```python
from build123d import *

# Parameters (mm, degrees)
F1_DEPTH = 19
F3_D     = 9
F3_DEPTH = 30
F2_R     = 8.5
F2_R_2   = 7.5
F4_DEPTH = 10


with BuildPart() as f1:
    # F0 (on Front) → F1 (new body)
    with BuildSketch(Plane.XZ):
        Polygon((0, 10), (0, 0), (17, 0), align=None)
    extrude(amount=F1_DEPTH)

    # F3
    with Locations(Plane(origin=(4.37018, 0, 7.429306), x_dir=(0.861934, 0, -0.50702), z_dir=(0.50702, 0, 0.861934))):
        with Locations((4.79134, -9.5)):
            Hole(F3_D / 2, depth=F3_DEPTH)

    # F2 (on face) → F4 (join)
    with BuildSketch(Plane(origin=(4.37018, 0, 7.429306), x_dir=(0.861934, 0, -0.50702), z_dir=(0.50702, 0, 0.861934))):
        with Locations((4.79134, -9.5)):
            Circle(F2_R)
        with Locations((4.79134, -9.5)):
            Circle(F2_R_2, mode=Mode.SUBTRACT)
    extrude(amount=F4_DEPTH)


solid = f1.part
```
Design review of the part built by this model. Coordinates are the model's own, in mm. A direction names the side the tool comes from. Coordinates: 2 decimals unless noted, no trailing zeros. Write each loop counter-clockwise with the first axis right and the second up, starting at its lowest first coordinate (ties: lowest second). Pieces come first, ordered by that corner, then holes.
1) Add section A-A (y = -5.5). Write out the cut boundary in (x, z), plus the area to 3 significant figures.
2) Insertion check: pin 1 (1.5 mm diameter, centred on x = 18.5, z = 8.5, fed in from +Y); pin 2 (8 mm diameter, centred on y = -13.5, z = 15, fed in from -X); pin 3 (4 mm diameter, centred on x = 14, y = -10, fed in from +Z). Each pin has a flat end and moves straight along its axis. Give the tip position at first contact, or say it passes through.
3) Machinability: for faces 5 (the flat face through (5, 0, 3)), 6 (the flat face through (6.73, -0.92, 6.04)), which of the approach directions +Z, -Z, +X, -X, +Y, -Y give a long, thin tool a straight path to every point of the face, cutting with its end or side? Answer none if there is none.
4) Add section C-C (z = 2.25). State how many separate pieces and enclosed holes the cut face has, plus the area to 3 significant figures.
5) Mouldability with a two-part tool opening along Y and no side actions: class faces 1 (the flat face through (8.591, -14.395, 4.947)), 2 (the flat face through (12, -9, 0)), 3 (the flat face through (5, -19, 3)), 4 (the cylindrical face through (3.1, -8.15, 4.29)) as +Y half, -Y half, draft (parallel to the pull), parting line (faces both ways), or undercut.
6) Add section B-B (y = -12). Write out the cut boundary in (x, z) (3 decimals), plus the area to 3 significant figures.
7) To check wall thickness, follow L1, parallel to X at y = -8.5, z = 1.75 (3 decimals); L2, parallel to Y at x = 8.75, z = 6 (3 decimals); L3, parallel to X at y = -5.5, z = 3.25 (3 decimals). State the ranges of each line that lie inside material, in increasing order.
Check result:
1. outline: (0, 0) - (3.17, 0) - (6.72, 6.05) - (3.03, 8.22) - (8.1, 16.84) - (7.11, 17.42) - (2.04, 8.8) - (0, 10) - close; (7.95, 0) - (17, 0) - (14.96, 1.2) - (20.03, 9.82) - (19.04, 10.4) - (13.97, 1.78) - (10.28, 3.95) - close
1. area: 84.2 mm2
2. pin 1: stops at y = -3.58
2. pin 2: stops at x = 2.76
2. pin 3: stops at z = 3.01
3. face 5: +Z, -Z, +X, -X, +Y
3. face 6: none
4. separate pieces: 1
4. enclosed holes: 2
4. area: 192 mm2
5. face 1: undercut
5. face 2: draft
5. face 3: -Y half
5. face 4: undercut
6. outline: (0, 0) - (1.218, 0) - (5.275, 6.897) - (2.405, 8.585) - (7.475, 17.205) - (6.568, 17.738) - (1.498, 9.119) - (0, 10) - close; (9.9, 0) - (17, 0) - (15.502, 0.881) - (20.573, 9.5) - (19.665, 10.034) - (14.595, 1.415) - (11.725, 3.103) - close
6. area: 62.6 mm2
7. L1: x = 0 to 1.498, 11.679 to 14.025, 15.212 to 16.381
7. L2: y = -17.995 to -16.994, -2.006 to -1.005
7. L3: x = 0 to 5.079, 9.862 to 11.475, 14.831 to 16.172
